Can you work these out from the model? Positions are in its coordinate system, mm. Face numbers are marked on the shaded views. A direction names the side the tool comes from. Coordinates: 2 decimals unless noted, no trailing zeros. Order: outer loops, then holes, each group sorted by start corner. A loop starts at its lowest first (then second) coordinate and runs counter-clockwise, first axis right, second up. Notation, with made-up numbers: (26.5, 46.25) -> (36.5, 46.25) arc R20 cw to (36.5, 71.25) -> close; hole circle Ø2 at (18.25, -36.75). An arc over 180 degrees is marked (long way). Return JSON: item names as keys, results as strings. Group by question number.
1) If we section it at C-C, the plane z = 0: State how many separate pieces and enclosed holes the cut face has, then the cut area to 3 significant figures.
2) If I drill on probe 1 along Y at (x, z) = (27, -39) (3 decimals); probe 2 along X at (y, z) = (-0.75, 54); probe 3 along X at (y, z) = (-2.5, 50), over which ranges is the centre line in solid material (lowest first)? Write a range as from..to.
3) For pin 1 (4 mm diameter, centred on x = 15.5, y = -8, fed in from -Z); pin 2 (4 mm diameter, centred on y = -21.5, z = -10.5, fed in from -X); pin 3 (4 mm diameter, centred on y = -21, z = 8.5, fed in from +X); pin 4 (3 mm diameter, centred on x = -51.69, z = 29.84, fed in from +Y), each with a flat end and sliding along its axis, tell me the tip position at first contact or that it passes through.
4) If we section it at B-B, the plane x = 59.69: Please give me the cut outline in (y, z).
5) If we section it at A-A, the plane z = -59.69: Please give me the cut outline in (x, y).
6) For the marked faces 1 and 2, which set-ups out of +Z, -Z, +X, -X, +Y, -Y let a thin tool reach every point of the face, with its end or its side?
from build123d import *

# Parameters (mm, degrees)
SKETCH1_W           = 26.67
SKETCH1_H           = 6.35
SKETCH2_R           = 49.53
SKETCH2_R_2         = 43.18
BOSS_EXTRUDE1_DEPTH = 19.05
SKETCH3_W           = 3.175
SKETCH3_H           = 2.116666667
SKETCH3_H_2         = 2.116666666
SKETCH4_R           = 2.54
CUT_EXTRUDE1_DEPTH  = 26.4
CIRPATTERN1_COUNT   = 12


with BuildPart() as part:
    # Sketch1 → Revolve1 (revolve)
    with BuildSketch(Plane.XY):
        with Locations((56.515, -3.175)):
            Rectangle(SKETCH1_W, SKETCH1_H)
    revolve(axis=Axis((0, -127, 0), (0, 1, 0)))

    # Sketch2 → Boss-Extrude1 (add)
    with BuildSketch(Plane.XZ.offset(6.35)):
        Circle(SKETCH2_R)
        Circle(SKETCH2_R_2, mode=Mode.SUBTRACT)
    extrude(amount=BOSS_EXTRUDE1_DEPTH)

    # Sketch3 → Cut-Revolve1 (revolve, cut)
    with BuildSketch(Plane.XY):
        with Locations((47.9425, -21.166666666)):
            Rectangle(SKETCH3_W, SKETCH3_H)
        with Locations((47.9425, -15.875)):
            Rectangle(SKETCH3_W, SKETCH3_H_2)
        with Locations((47.9425, -10.583333334)):
            Rectangle(SKETCH3_W, SKETCH3_H)
    revolve(axis=Axis((0, 0, 0), (0, -1, 0)), mode=Mode.SUBTRACT)

    # Sketch4 → Cut-Extrude1 (cut, through all)
    with BuildSketch(Plane(origin=(0, 0, 0), x_dir=(1, 0, 0), z_dir=(0, 1, 0))):
        with Locations((-59.69, 0)):
            Circle(SKETCH4_R)
    cut_extrude1 = extrude(amount=-CUT_EXTRUDE1_DEPTH, mode=Mode.SUBTRACT)

    # CirPattern1: Cut-Extrude1 ×12 about axis
    cirpattern1_axis = Axis((0, 0, 0), (0, 1, 0))
    for i in range(1, CIRPATTERN1_COUNT):
        add(cut_extrude1.rotate(cirpattern1_axis, i * 360 / CIRPATTERN1_COUNT), mode=Mode.SUBTRACT)


solid = part.part
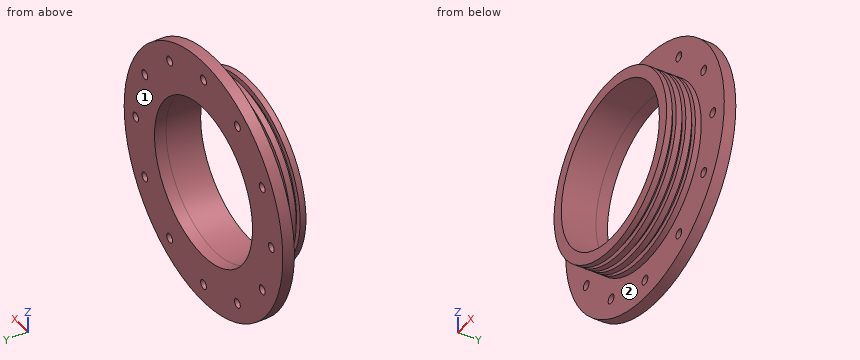
Result sheet:
{
 "1": {"separate pieces": "4", "enclosed holes": "0", "area": "476 mm2"},
 "2": {"probe 1": "y = -25.4..-22.225, -20.108..-16.933, -14.817..-11.642, -9.525..0", "probe 2": "x = -44.31..-30.91, -28.78..28.78, 30.91..44.31", "probe 3": "x = -48.78..-31.74, -27.95..27.95, 31.74..48.78"},
 "3": {"pin 1": "stops at z = -68.36", "pin 2": "stops at x = -48.77", "pin 3": "stops at x = 49.07", "pin 4": "passes through"},
 "4": {"outline": "(-6.35, -36.28) -> (0, -36.28) -> (0, -2.54) -> (-6.35, -2.54) -> close; (-6.35, 2.54) -> (0, 2.54) -> (0, 36.28) -> (-6.35, 36.28) -> close"},
 "5": {"outline": "(-36.28, -6.35) -> (-2.54, -6.35) -> (-2.54, 0) -> (-36.28, 0) -> close; (2.54, -6.35) -> (36.28, -6.35) -> (36.28, 0) -> (2.54, 0) -> close"},
 "6": {"face 1": "+Z, -Z, +X, -X, +Y", "face 2": "-Y"}
}
